Read the model definition and answer for the solid it produces. Units are mm, in the model's axes. A direction names the side the tool comes from. Round coordinates to 2 decimals unless told otherwise and drop trailing zeros. Order: outer loops, then holes, each group sorted by start corner. A loop starts at its lowest first (then second) coordinate and runs counter-clockwise, first axis right, second up. Notation, with made-up numbers: (33.5, -29) - (78.5, -29) arc R20 cw to (78.5, -4) - close; hole circle Ø10 at (8.5, 81). An arc over 180 degrees is marked (long way). One line per question, with ' | ' between items. Start each with the question number.
1) The part is cut by section A-A, the plane x = -27.5. Give the vertices of the cut face in (y, z), plus the area to 3 significant figures.
2) The mould has two halves that part along Z. Classify faces 1 (the cylindrical face through (29, 63, 64)), 2 (the flat face through (-1, 103, 65)), 3 (the flat face through (-62.5, 103, -1)): pulls with the +Z half, pulls with the -Z half, needs draft (parallel to the pull), parting line crosses it, or undercut.
3) Straight lines are drawn through the part: line 1 (Y direction, x = -27, z = -63); line 2 (X direction, y = 2, z = 56); line 3 (Y direction, x = -27.5, z = -63.15). For each, find the intervals that lie inside material, in ascending order. Write a range as from..to.
4) The part is cut by section D-D, the plane x = 6.5. Give the vertices of the cut face in (y, z).
5) The part is cut by section B-B, the plane y = 65. Give the vertices of the cut face in (x, z).
6) Flat-ended cylindrical pins translate along their axes: pin 1 (4.5 mm diameter, centred on x = -56.25, z = 56.25, fed in from +Y); pin 2 (6 mm diameter, centred on y = 168.75, z = 56.25, fed in from +X). Find the tip coordinate at first contact, or state that the pin passes through.
7) The part is cut by section C-C, the plane z = 8. Give the vertices of the cut face in (x, y), plus the area to 4 significant figures.
8) For faces 4 (the cylindrical face through (27.83, 170.52, 63.77)), 5 (the flat face through (-60, 204, 0)), determine the directions among +Z, -Z, +X, -X, +Y, -Y from which every point of the face is accessible in a straight line to the end or side of a thin tool.
Autodesk Inventor part; units mm, degrees
ref_plane "YZ Plane" through (0, 0, 0) normal (1, 0, 0) x (0, 1, 0)
ref_plane "XZ Plane" through (0, 0, 0) normal (0, 1, 0) x (-1, 0, 0)
ref_plane "XY Plane" through (0, 0, 0) normal (0, 0, 1) x (1, 0, 0)
sketch "Sketch1" plane through (0, 0, 0) normal (0, 1, 0) x (-1, 0, 0)
  line L0 (65, 65) -> (-65, 65)
  line L1 (-65, 65) -> (-65, -65)
  line L2 (-65, -65) -> (65, -65)
  line L3 (65, -65) -> (65, 65)
  line L4 (65, 65) -> (-65, -65) construction
  line L5 (-65, 65) -> (65, -65) construction
  circle A0 centre (-56.25, 56.25) radius 2.5
  line L6 (0, 15.2849) -> (0, -21.0051)
  line L7 (0, -21.0051) -> (-20.003, 0)
  line L8 (-20.003, 0) -> (15.941, 0)
  circle A1 centre (56.25, 56.25) radius 2.5
  circle A2 centre (-56.25, -56.25) radius 2.5
  circle A3 centre (56.25, -56.25) radius 2.5
  point P0 (0, 0)
  point P1 (0, 0)
  dimension "d0" = 130
  dimension "d1" = 130
  dimension "d2" = 5
  dimension "d3" = 8.75
extrude "Extrusion1" add sketch "Sketch1" along normal blind 4 contours L3 L2 L1 L0 | L6 L7 L8
sketch "Sketch2" plane through (0, 4, 0) normal (0, 1, 0) x (1, 0, 0)
  line L0 (-62.5, -62.5) -> (62.5, -62.5)
  line L1 (62.5, -62.5) -> (62.5, 62.5)
  line L2 (62.5, 62.5) -> (-62.5, 62.5)
  line L3 (-62.5, 62.5) -> (-62.5, -62.5)
  line L4 (-62.5, -62.5) -> (62.5, 62.5) construction
  line L5 (62.5, -62.5) -> (-62.5, 62.5) construction
  line L6 (-65, 65) -> (-65, -65)
  line L7 (65, 65) -> (-65, 65)
  line L8 (-65, -65) -> (65, -65)
  line L9 (65, -65) -> (65, 65)
  line L10 (65, 65) -> (-65, 65)
  line L11 (-65, 65) -> (-65, -65)
  line L12 (-65, -65) -> (65, 65) construction
  line L13 (65, -65) -> (-65, 65) construction
  line L14 (62.5, -62.5) -> (65, -62.5)
  line L15 (62.5, 62.5) -> (65, 62.5)
  point P0 (0, 0)
  dimension "d6" = 2.5
  dimension "d7" = 2.5
extrude "Extrusion2" add sketch "Sketch2" along normal blind 204 contours L0 L14 L9 L8 L6 L7 L15 L2 L3
sketch "Sketch3" plane through (0, 208, 0) normal (0, 1, 0) x (1, 0, 0)
  line L0 (-65, 65) -> (-65, -65)
  line L1 (-65, -65) -> (-47.5, -65)
  line L2 (-47.5, -65) -> (-47.5, -47.5)
  line L3 (-47.5, -47.5) -> (-65, -47.5)
  line L4 (-65, -47.5) -> (-65, -65)
  line L5 (-65, 65) -> (-47.5, 65)
  line L6 (-47.5, 65) -> (-47.5, 47.5)
  line L7 (-47.5, 47.5) -> (-65, 47.5)
  line L8 (-65, 47.5) -> (-65, 65)
  line L9 (-65, -65) -> (65, -65)
  line L10 (65, -65) -> (47.5, -65)
  line L11 (47.5, -65) -> (47.5, -47.5)
  line L12 (47.5, -47.5) -> (65, -47.5)
  line L13 (65, -47.5) -> (65, -65)
  line L14 (65, 65) -> (-65, 65)
  line L15 (65, 65) -> (47.5, 65)
  line L16 (47.5, 65) -> (47.5, 47.5)
  line L17 (47.5, 47.5) -> (65, 47.5)
  line L18 (65, 47.5) -> (65, 65)
  circle A0 centre (56.25, -56.25) radius 2.5
  circle A1 centre (56.25, 56.25) radius 2.5
  circle A2 centre (56.25, 56.25) radius 2.5
  circle A3 centre (-56.25, 56.25) radius 2.5
  circle A4 centre (-56.25, -56.25) radius 2.5
  circle A5 centre (-56.25, -56.25) radius 2.5
  line L19 (-47.5, -56.25) -> (47.5, -56.25)
  line L20 (-56.25, -47.5) -> (-56.25, 47.5)
  line L21 (-47.5, 56.25) -> (47.5, 56.25)
  point P0 (0, 0)
  point P1 (56.25, -65)
  dimension "d10" = 17.5
  dimension "d11" = 17.5
  dimension "d12" = 17.5
  dimension "d13" = 17.5
  dimension "d14" = 17.5
  dimension "d15" = 17.5
  dimension "d16" = 17.5
  dimension "d17" = 17.5
  dimension "d18" = 5
  dimension "d19" = 5
  dimension "d20" = 5
  dimension "d21" = 5
extrude "Extrusion3" add sketch "Sketch3" against normal blind 4
sketch "Sketch4" plane through (-65, 0, -65) normal (-1, 0, 0) x (0, 0, 1)
  circle A0 centre (8.75, 168.75) radius 2.5
  circle A1 centre (121.25, 168.75) radius 2.5
  line L0 (0, 208) -> (130, 208)
  line L1 (0, 0) -> (0, 208)
  line L2 (130, 0) -> (130, 208)
  point P0 (65, 0)
  dimension "d24" = 5
  dimension "d25" = 5
  dimension "d26" = 39.25
  dimension "d27" = 39.25
  dimension "d28" = 8.75
  dimension "d29" = 8.75
extrude "Extrusion4" cut sketch "Sketch4" against normal through all
sketch "Sketch7" plane through (-65, 0, 65) normal (0, 0, 1) x (1, 0, 0)
  circle A0 centre (37.5, 173) radius 2.5
  circle A1 centre (92.5, 173) radius 2.5
  circle A2 centre (37.5, 65) radius 2.5
  circle A3 centre (92.5, 65) radius 2.5
  line L0 (0, 208) -> (130, 208)
  line L1 (130, 0) -> (130, 208)
  line L2 (0, 0) -> (130, 0)
  point P0 (65, 0)
  dimension "d47" = 5
  dimension "d48" = 5
  dimension "d49" = 5
  dimension "d50" = 5
  dimension "d51" = 55
  dimension "d52" = 55
  dimension "d53" = 0
  dimension "d54" = 35
  dimension "d55" = 0
  dimension "d56" = 37.5
  dimension "d57" = 37.5
  dimension "d58" = 65
sketch "Sketch5" plane through (65, 0, -65) normal (0, 0, -1) x (-1, 0, 0)
  circle A0 centre (37.5, 173) radius 2.5
  circle A1 centre (92.5, 173) radius 2.5
  circle A2 centre (37.5, 65) radius 2.5
  circle A3 centre (92.5, 65) radius 2.5
  line L0 (130, 0) -> (130, 208)
  line L1 (0, 208) -> (130, 208)
  line L2 (0, 0) -> (130, 0)
  point P0 (65, 0)
  dimension "d32" = 5
  dimension "d33" = 5
  dimension "d34" = 5
  dimension "d35" = 5
  dimension "d36" = 55
  dimension "d37" = 55
  dimension "d38" = 0
  dimension "d39" = 37.5
  dimension "d40" = 37.5
  dimension "d41" = 35
  dimension "d42" = 65
  dimension "d43" = 35
extrude "Extrusion5" cut sketch "Sketch5" against normal blind 10
sketch "Sketch6" plane through (65, 0, -65) normal (0, 0, -1) x (-1, 0, 0)
  point P0 (65, 0)
mirror "Mirror1" about plane through (0, 0, 0) normal (0, 0, 1) of "Extrusion5"
Values:
1) outline: (0, -65) - (62.5, -65) - (62.5, -62.5) - (4, -62.5) - (4, 62.5) - (62.5, 62.5) - (62.5, 65) - (0, 65) - close; (67.5, -65) - (170.5, -65) - (170.5, -62.5) - (67.5, -62.5) - close; (67.5, 62.5) - (170.5, 62.5) - (170.5, 65) - (67.5, 65) - close; (175.5, -65) - (208, -65) - (208, -56.25) - (204, -56.25) - (204, -62.5) - (175.5, -62.5) - close; (175.5, 62.5) - (204, 62.5) - (204, 56.25) - (208, 56.25) - (208, 65) - (175.5, 65) - close | area: 1,540 mm^2
2) face 1: needs draft | face 2: pulls with the +Z half | face 3: undercut
3) line 1: y = 0..62.55, 67.45..170.55, 175.45..208 | line 2: x = -65..-58.74, -53.76..53.76, 58.74..65 | line 3: y = 0..62.5, 67.5..170.5, 175.5..208
4) outline: (0, -65) - (208, -65) - (208, -56.25) - (204, -56.25) - (204, -62.5) - (4, -62.5) - (4, 62.5) - (204, 62.5) - (204, 56.25) - (208, 56.25) - (208, 65) - (0, 65) - close
5) outline: (-65, -65) - (-30, -65) - (-30, -62.5) - (-62.5, -62.5) - (-62.5, 62.5) - (-30, 62.5) - (-30, 65) - (-65, 65) - close; (-25, -65) - (25, -65) - (25, -62.5) - (-25, -62.5) - close; (-25, 62.5) - (25, 62.5) - (25, 65) - (-25, 65) - close; (30, -65) - (65, -65) - (65, -62.5) - (30, -62.5) - close; (30, 62.5) - (65, 62.5) - (65, 65) - (30, 65) - close
6) pin 1: passes through | pin 2: stops at x = -62.5
7) outline: (-65, 0) - (65, 0) - (65, 4) - (-62.5, 4) - (-62.5, 204) - (-56.25, 204) - (-56.25, 208) - (-65, 208) - close | area: 1,055 mm^2
8) face 4: +Z, -Z | face 5: +X
